```python
from build123d import *

# Parameters (mm, degrees)
F3_SIZE = 1.27
F4_SIZE = 1.27


with BuildPart() as f2:
    # F0 (on Front) → F2 (revolve)
    with BuildSketch(Plane.XZ):
        Polygon((-8.382, 0), (-8.382, 45.466), (-14.732, 45.466), (-19.05, 10.922), (-19.05, -45.466), (-8.382, -45.466), align=None)
    revolve(axis=Axis((0, 0, 0.149863), (0, 0, -1)))

    # F3
    f3_edges = [f2.edges().sort_by_distance(p)[0] for p in [
        (8.382, 0, 45.466),
    ]]
    chamfer(f3_edges, length=F3_SIZE)

    # F4
    f4_edges = [f2.edges().sort_by_distance(p)[0] for p in [
        (8.382, 0, -45.466),
    ]]
    chamfer(f4_edges, length=F4_SIZE)


solid = f2.part
```
Model file for the job. Use its own axes, mm. Give positions to 0.01 mm unless a question says otherwise; leave off trailing zeros. Write each loop counter-clockwise with the first axis right and the second up, starting at its lowest first coordinate (ties: lowest second). Pieces come first, ordered by that corner, then holes. Notation, with made-up numbers: (89.25, -13.75) -> (131.25, -13.75) arc R9 cw to (131.25, -6.75) -> close; hole circle Ø5 at (-21.75, -25.5). An arc over 180 degrees is marked (long way). Use CSV: the item, a comma, the result in double quotes. Start each with the question number.
1) Cut at C-C on z = -2. List the corners of the cut face in (x, y), plus the area to 3 significant figures.
2) Pin check, flat tips, straight feed: P1, Ø1.5, axis at y = -14.5, z = -27, coming from the +X side; P2, Ø5, axis at y = -13.5, z = 5.5, coming from the -X side; P3, Ø5, axis at y = -13.5, z = -4.5, coming from the +X side. Stop position of each tip, or through.
3) Cut at A-A on y = 0. List the corners of the cut face in (x, z), plus the area to 3 significant figures.
4) Two-plate mould, pull along Y, no slides. Class faces 1 (the cylindrical face through (-8, 2.5, 0.6)), 2 (the cylindrical face through (15.12, -11.59, -17.67)), 3 (the flat face through (5, 9, -45.466)): released by +Y, released by -Y, zero draft, split by the parting line, or undercut.
5) Drill centre lines: L1, parallel to Y at x = 0, z = -13.5; L2, parallel to Y at x = -1.5, z = -27.5; L3, parallel to X at y = -2.5, z = -13. Where is each one in solid material? Low to high.
Final values:
1,outline,"circle Ø38.1 at (0, 0); hole circle Ø16.76 at (0, 0)"
1,area,"919 mm2"
2,P1,"stops at x = 13.18"
2,P2,"stops at x = -15.55"
2,P3,"stops at x = 15.55"
3,outline,"(-19.05, -45.47) -> (-9.65, -45.47) -> (-8.38, -44.2) -> (-8.38, 44.2) -> (-9.65, 45.47) -> (-14.73, 45.47) -> (-19.05, 10.92) -> close; (8.38, -44.2) -> (9.65, -45.47) -> (19.05, -45.47) -> (19.05, 10.92) -> (14.73, 45.47) -> (9.65, 45.47) -> (8.38, 44.2) -> close"
3,area,"1,790 mm2"
4,face 1,"undercut"
4,face 2,"split by the parting line"
4,face 3,"zero draft"
5,L1,"y = -19.05 to -8.38, 8.38 to 19.05"
5,L2,"y = -18.99 to -8.25, 8.25 to 18.99"
5,L3,"x = -18.89 to -8, 8 to 18.89"
